from build123d import *

# Parameters (mm, degrees)
SKETCH1_W           = 25
SKETCH1_H           = 25
SKETCH1_W_2         = 20.25
SKETCH1_H_2         = 20.25
BOSS_EXTRUDE1_DEPTH = 5
SKETCH2_R           = 2.625
SKETCH2_W           = 20.25
SKETCH2_H           = 20.25
BOSS_EXTRUDE2_DEPTH = 5
SKETCH3_W           = 25
SKETCH3_H           = 25
SKETCH3_W_2         = 20.25
SKETCH3_H_2         = 20.25
BOSS_EXTRUDE3_DEPTH = 20
SKETCH4_R           = 2.625
CUT_EXTRUDE1_DEPTH  = 38.5
SKETCH5_R           = 2.625
CUT_EXTRUDE2_DEPTH  = 38.5
FILLET1_R           = 2


with BuildPart() as part:
    # Sketch1 → Boss-Extrude1 (new body, symmetric)
    with BuildSketch(Plane.XY):
        Rectangle(SKETCH1_W, SKETCH1_H)
        Rectangle(SKETCH1_W_2, SKETCH1_H_2, mode=Mode.SUBTRACT)
    extrude(amount=BOSS_EXTRUDE1_DEPTH, both=True)

    # Sketch2 → Boss-Extrude2 (add, symmetric)
    with BuildSketch(Plane.XY):
        Polygon((-25, 0), (0, 25), (25, 0), (0, -25), align=None)
        with Locations((0, 19.75)):
            Circle(SKETCH2_R, mode=Mode.SUBTRACT)
        with Locations((19.75, 0)):
            Circle(SKETCH2_R, mode=Mode.SUBTRACT)
        with Locations((0, -19.75)):
            Circle(SKETCH2_R, mode=Mode.SUBTRACT)
        with Locations((-19.75, 0)):
            Circle(SKETCH2_R, mode=Mode.SUBTRACT)
        Rectangle(SKETCH2_W, SKETCH2_H, mode=Mode.SUBTRACT)
    extrude(amount=BOSS_EXTRUDE2_DEPTH, both=True)

    # Sketch3 → Boss-Extrude3 (add)
    with BuildSketch(Plane.XY.offset(5)):
        Rectangle(SKETCH3_W, SKETCH3_H)
        Rectangle(SKETCH3_W_2, SKETCH3_H_2, mode=Mode.SUBTRACT)
    extrude(amount=BOSS_EXTRUDE3_DEPTH)

    # Sketch4 → Cut-Extrude1 (cut, through all)
    with BuildSketch(Plane(origin=(0, 12.5, 0), x_dir=(1, 0, 0), z_dir=(0, 1, 0))):
        with Locations((0, -15)):
            Circle(SKETCH4_R)
    extrude(amount=-CUT_EXTRUDE1_DEPTH, mode=Mode.SUBTRACT)

    # Sketch5 → Cut-Extrude2 (cut, through all)
    with BuildSketch(Plane(origin=(12.5, 0, 0), x_dir=(0, 0, -1), z_dir=(1, 0, 0))):
        with Locations((-15, 0)):
            Circle(SKETCH5_R)
    extrude(amount=-CUT_EXTRUDE2_DEPTH, mode=Mode.SUBTRACT)

    # Fillet1
    fillet1_edges = [part.edges().sort_by_distance(p)[0] for p in [
        (0, -25, 0),
        (25, 0, 0),
        (0, 25, 0),
        (-25, 0, 0),
    ]]
    fillet(fillet1_edges, radius=FILLET1_R)


solid = part.part
Geometry: final body of the model. Coordinates: model frame, mm. A direction names the side the tool comes from. Give positions to 0.01 mm unless a question says otherwise; leave off trailing zeros. Write each loop counter-clockwise with the first axis right and the second up, starting at its lowest first coordinate (ties: lowest second). Pieces come first, ordered by that corner, then holes. Notation, with made-up numbers: M 25.5,1.25 L 32.5,1.25 A18 ccw 32.5,29.25 Z; hole C 33.5,-18 d6. An arc over 180 degrees is marked long. Answer in a Markdown table with one row per item. Add a question column.
(1) Ray query, line 1 (Y direction, x = -7, z = 18.25) (3 decimals); line 2 (Y direction, x = 0, z = 1.5) (3 decimals); line 3 (X direction, y = 1, z = 3.5) (3 decimals). Return the intervals inside material, ascending.
(2) Section A-A on x = -7. Return loops of the section in (y, z) (3 decimals).
(3) Section B-B on y = 19.75. Return loops of the section in (x, z) (3 decimals), and give its area (3 significant figures).
(4) First-contact query: pin 1 (6 mm diameter, centred on x = 0, y = 19.75, fed in from +Z); pin 2 (12 mm diameter, centred on x = 2.5, z = 17.5, fed in from -Y); pin 3 (1.5 mm diameter, centred on y = 1, z = 18, fed in from -X). Flat tips, straight axial feed; report the tip coordinate or a pass-through.
(5) Section D-D on x = 0. Return loops of the section in (y, z) (3 decimals), and give its area (3 significant figures).
(6) Section C-C on z = -2.25. Return loops of the section in (x, y) (3 decimals), and give its area (3 significant figures).
(7) Mould query, pull axis Z, two halves, no side actions, for faces 1 (the flat face through (16, 0, 5)), 2 (the flat face through (-3, -12.5, 15)), 3 (the cylindrical face through (1.21, -11.3, 17.33)), 4 (the cylindrical face through (11.329, 0.115, 17.622)). Classes: +Z half, -Z half, draft (parallel to the pull), parting line (faces both ways), or undercut.
(8) Reachability of faces 5 (the flat face through (0, -16, 5)), 6 (the flat face through (0, 16, 5)), 7 (the flat face through (0, -10.125, 10)) from +Z, -Z, +X, -X, +Y, -Y: full face, straight path, thin tool, end or side. Return the list, or none.
Result set:
| question | item | result |
|---|---|---|
| 1 | line 1 | y = -12.5 to -10.125, 10.125 to 12.5 |
| 1 | line 2 | y = -24.172 to -22.375, -17.125 to -10.125, 10.125 to 17.125, 22.375 to 24.172 |
| 1 | line 3 | x = -23.904 to -22.177, -17.323 to -10.125, 10.125 to 17.323, 22.177 to 23.904 |
| 2 | outline | M -18,-5 L -10.125,-5 L -10.125,25 L -12.5,25 L -12.5,5 L -18,5 Z; M 10.125,-5 L 18,-5 L 18,5 L 12.5,5 L 12.5,25 L 10.125,25 Z |
| 3 | outline | M -5.25,-5 L -2.625,-5 L -2.625,5 L -5.25,5 Z; M 2.625,-5 L 5.25,-5 L 5.25,5 L 2.625,5 Z |
| 3 | area | 52.5 mm^2 |
| 4 | pin 1 | stops at z = 5 |
| 4 | pin 2 | stops at y = -12.5 |
| 4 | pin 3 | stops at x = -12.5 |
| 5 | outline | M -24.172,-5 L -22.375,-5 L -22.375,5 L -24.172,5 Z; M -17.125,-5 L -10.125,-5 L -10.125,12.375 L -12.5,12.375 L -12.5,5 L -17.125,5 Z; M -12.5,17.625 L -10.125,17.625 L -10.125,25 L -12.5,25 Z; M 10.125,-5 L 17.125,-5 L 17.125,5 L 12.5,5 L 12.5,12.375 L 10.125,12.375 Z; M 10.125,17.625 L 12.5,17.625 L 12.5,25 L 10.125,25 Z; M 22.375,-5 L 24.172,-5 L 24.172,5 L 22.375,5 Z |
| 5 | area | 246 mm^2 |
| 6 | outline | M -23.586,-1.414 L -1.414,-23.586 A2 ccw 1.414,-23.586 L 23.586,-1.414 A2 ccw 23.586,1.414 L 1.414,23.586 A2 ccw -1.414,23.586 L -23.586,1.414 A2 ccw Z; hole C -19.75,0 d5.25; hole M -10.125,-10.125 L 10.125,-10.125 L 10.125,10.125 L -10.125,10.125 Z; hole C 0,-19.75 d5.25; hole C 0,19.75 d5.25; hole C 19.75,0 d5.25 |
| 6 | area | 750 mm^2 |
| 7 | face 1 | +Z half |
| 7 | face 2 | draft |
| 7 | face 3 | undercut |
| 7 | face 4 | undercut |
| 8 | face 5 | +Z, +X, -X, -Y |
| 8 | face 6 | +Z, +X, -X, +Y |
| 8 | face 7 | +Z, -Z |
